Design review of the part built by this model. Coordinates are the model's own, in mm. Face numbers are marked on the shaded views. A direction names the side the tool comes from. Give positions to 0.01 mm unless a question says otherwise; leave off trailing zeros. Loops run counter-clockwise (first coordinate to the right, second up) from the corner with the lowest first, then second, coordinate; pieces in that order, holes last. Notation, with made-up numbers: (36.5, -29) - (66.5, -29) arc R13 cw to (66.5, -13) - close; hole circle Ø3 at (64, 76.25). An arc over 180 degrees is marked (long way). Put each result on its own line as item: value. Start each with the question number.
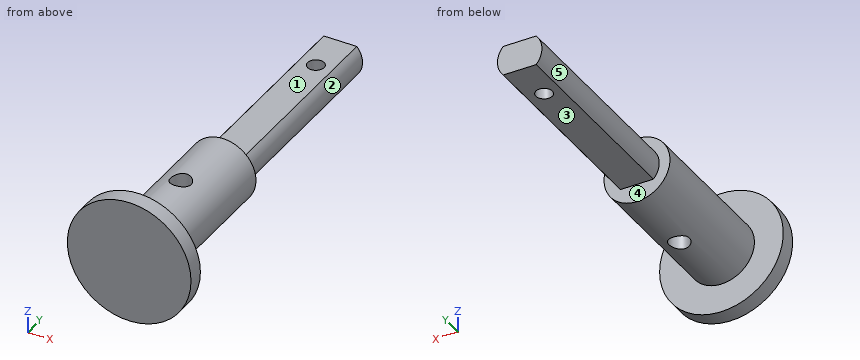
```python
from build123d import *

# Parameters (mm, degrees)
SKETCH1_R               = 7.5
SKETCH1_R_2             = 4
BOSS_EXTRUDE1_DEPTH     = 2
SKETCH1_2_R             = 4
BOSS_EXTRUDE2_DEPTH     = 45
SKETCH2_R               = 4.5
CUT_EXTRUDE1_DEPTH      = 25
SKETCH3_R               = 1
SKETCH3_R_2             = 1.25
CUT_EXTRUDE2_DEPTH      = 25
CUT_EXTRUDE2_DEPTH_BACK = 25


with BuildPart() as part:
    # Sketch1 → Boss-Extrude1 (new body)
    with BuildSketch(Plane(origin=(0, 0, 0), x_dir=(1, 0, 0), z_dir=(0, 1, 0))):
        Circle(SKETCH1_R)
        Circle(SKETCH1_R_2, mode=Mode.SUBTRACT)
    extrude(amount=BOSS_EXTRUDE1_DEPTH)

    # Sketch1_2 → Boss-Extrude2 (add)
    with BuildSketch(Plane(origin=(0, 0, 0), x_dir=(1, 0, 0), z_dir=(0, 1, 0))):
        Circle(SKETCH1_2_R)
    extrude(amount=BOSS_EXTRUDE2_DEPTH)

    # Sketch2 → Cut-Extrude1 (cut)
    with BuildSketch(Plane(origin=(0, 45, 0), x_dir=(1, 0, 0), z_dir=(0, 1, 0))):
        Circle(SKETCH2_R)
        with BuildLine():
            Line((-2, 1.811376185), (2, 1.811376185))
            ThreePointArc((2, 1.811376185), (2.698348325, 0), (2, -1.811376185))
            Line((2, -1.811376185), (-2, -1.811376185))
            ThreePointArc((-2, -1.811376185), (-2.698348325, 0), (-2, 1.811376185))
        make_face(mode=Mode.SUBTRACT)
    extrude(amount=-CUT_EXTRUDE1_DEPTH, mode=Mode.SUBTRACT)

    # Sketch3 → Cut-Extrude2 (cut, two sides)
    with BuildSketch(Plane(origin=(0, 0, -1.811376185), x_dir=(-1, 0, 0), z_dir=(0, 0, -1))) as cut_extrude2_sk:
        with Locations((0, 39.794309812)):
            Circle(SKETCH3_R)
        with Locations((0, 11)):
            Circle(SKETCH3_R_2)
    extrude(amount=CUT_EXTRUDE2_DEPTH, mode=Mode.SUBTRACT)
    extrude(cut_extrude2_sk.sketch, amount=-CUT_EXTRUDE2_DEPTH_BACK, mode=Mode.SUBTRACT)


solid = part.part
```
Item 1: Consider section D-D (y = 31). State the section outline as (x, z) points.
Item 2: Machinability: for the marked faces 1, 2, 3, 4 and 5, which of the approach directions +Z, -Z, +X, -X, +Y, -Y give a long, thin tool a straight path to every point of the face, cutting with its end or side? Answer none if there is none.
Item 3: For P1, Ø3, axis at x = 0, y = 11, coming from the +Z side; P2, Ø1.5, axis at x = 0, y = 11, coming from the +Z side; P3, Ø1.5, axis at y = 33.5, z = -1, coming from the -X side; P4, Ø1.5, axis at x = 1, y = 7, coming from the -Z side, all flat-tipped, find the tip position at first contact; note any pin that passes through.
Item 4: For L1, parallel to Y at x = 0, z = 0.45; L2, parallel to Y at x = 0, z = -3; L3, parallel to X at y = 11, z = 0.2 (3 decimals), list the stretches that pass through material, from the lowest coordinate up. Write a range as from..to.
Item 5: Consider section C-C (z = 2.25). State the section outline as (x, y) points.
Item 6: Consider section A-A (x = 0). State the section outline as (y, z) points.
Item 7: Consider section B-B (z = 0). State the section outline as (x, y) points, plus the area to 3 significant figures.
Geometry says:
1. outline: (-2, -1.81) - (2, -1.81) arc R2.7 ccw to (2, 1.81) - (-2, 1.81) arc R2.7 ccw to start
2. face 1: +Z, +X, -X, +Y
2. face 2: +X, +Y
2. face 3: -Z, +X, -X, +Y
2. face 4: +Y
2. face 5: -X, +Y
3. P1: stops at z = 4
3. P2: passes through
3. P3: stops at x = -2.69
3. P4: stops at z = -3.99
4. L1: y = 0..9.75, 12.25..38.79, 40.79..45
4. L2: y = 0..9.75, 12.25..20
4. L3: x = -3.995..-1.25, 1.25..3.995
5. outline: (-7.15, 0) - (7.15, 0) - (7.15, 2) - (3.31, 2) - (3.31, 20) - (-3.31, 20) - (-3.31, 2) - (-7.15, 2) - close; hole circle Ø2.5 at (0, 11)
6. outline: (0, -7.5) - (2, -7.5) - (2, -4) - (9.75, -4) - (9.75, 4) - (2, 4) - (2, 7.5) - (0, 7.5) - close; (12.25, -4) - (20, -4) - (20, -1.81) - (38.79, -1.81) - (38.79, 1.81) - (20, 1.81) - (20, 4) - (12.25, 4) - close; (40.79, -1.81) - (45, -1.81) - (45, 1.81) - (40.79, 1.81) - close
7. outline: (-7.5, 0) - (7.5, 0) - (7.5, 2) - (4, 2) - (4, 20) - (2.7, 20) - (2.7, 45) - (-2.7, 45) - (-2.7, 20) - (-4, 20) - (-4, 2) - (-7.5, 2) - close; hole circle Ø2.5 at (0, 11); hole circle Ø2 at (0, 39.79)
7. area: 301 mm2
